Autodesk Inventor part; units mm, degrees
ref_plane "YZ Plane" through (0, 0, 0) normal (1, 0, 0) x (0, 1, 0)
ref_plane "XZ Plane" through (0, 0, 0) normal (0, 1, 0) x (-1, 0, 0)
ref_plane "XY Plane" through (0, 0, 0) normal (0, 0, 1) x (1, 0, 0)
sketch "Sketch1" plane through (0, 0, 0) normal (0, 0, 1) x (1, 0, 0)
  line L0 (-9, -10) -> (9, -10)
  line L1 (9, -10) -> (9, 10)
  line L2 (9, 10) -> (-9, 10)
  line L3 (-9, 10) -> (-9, -10)
  line L4 (-9, -10) -> (9, 10) construction
  line L5 (9, -10) -> (-9, 10) construction
  point P0 (0, 0)
  dimension "d0" = 18
  dimension "d1" = 20
extrude "Plate1" add sketch "Sketch1" along normal blind 2
sketch "Sketch2" plane through (9, -8.1451, -0.7479) normal (0, -0.9274452, 0.3739592) x (1, 0, 0)
  line L0 (-18, 0) -> (0, 0)
  line L1 (0, 0) -> (0, 12)
  line L2 (0, 12) -> (-18, 12)
  line L3 (-18, 12) -> (-18, 0)
edge flange "Flange1" height 12 angle 111.96 thickness 2 bend radius 2 thickness toward (0, -0.9274452, 0.3739592) relief tear relief width 2 relief depth 1 edges at (0, -10, 2) wall of the first edge with corners at (-9, -8.1451, -0.7479) (9, -8.1451, -0.7479) (9, -3.6576, 10.3814) (-9, -3.6576, 10.3814)
bend "Bend1"
corner "Corner1"
chamfer "Corner Chamfer1" distance 2 angle 45 4 edges at (-9, 10, 1) (9, 10, 1) (-9, -4.585, 10.7554) (9, -4.585, 10.7554)
equation "\"d3\" = BendReliefWidth"
equation "\"d4\" = BendReliefDepth"
equation "\"d5\" = MinimumRemnant"
equation "\"d6\" = BendRadius"
equation "\"d9\" = BendRadius"
equation "\"d10\" = CornerReliefSize"
equation "\"d11\" = GapSize"
equation "\"d12\" = JacobiRadiusSize"
equation "\"BendRadius\" = Thickness"
equation "\"BendReliefWidth\" = Thickness"
equation "\"BendReliefDepth\" = 0.5 * Thickness"
equation "\"CornerReliefSize\" = 4 * Thickness"
equation "\"MinimumRemnant\" = 2 * Thickness"
equation "\"TransitionRadius\" = BendRadius"
equation "\"JacobiRadiusSize\" = BendRadius"
equation "\"GapSize\" = Thickness"
equation "\"d2\" = BendRadius"
Here's how the part is built. I have some questions about the finished solid (model axes, mm). A direction names the side the tool comes from. Round coordinates to 2 decimals unless told otherwise and drop trailing zeros. Order: outer loops, then holes, each group sorted by start corner. A loop starts at its lowest first (then second) coordinate and runs counter-clockwise, first axis right, second up. Notation, with made-up numbers: M 81,77.25 L 137,77.25 A20 cw 137,83.25 Z; hole C -25.75,78.25 d5. An arc over 180 degrees is marked long. Answer in a Markdown table with one row per item.
Item 1: I'm going to push a flat-ended pin straight in: pin 1 (2 mm diameter, centred on x = -4.5, y = -0.5, fed in from +Z). Where does the tip first touch, or does it pass through?
A:
| item | result |
|---|---|
| pin 1 | stops at z = 2 |
Item 2: Thinking about a two-plate mould opening in Z: for faces 3 (the face through (0, 3, 0)), 4 (the face through (0.1, -4.57, 10.75)), 5 (the face through (0.126, -5.747, 2.904)), which applies, +Z half, -Z half, draft (parallel to the pull), parting line (faces both ways), or undercut?
A:
| item | result |
|---|---|
| face 3 | -Z half |
| face 4 | +Z half |
| face 5 | undercut |
Item 3: Imagine slicing it at A-A, the plane x = -1.25. Write out the boundary of the cut face in (y, z), and give its area (3 significant figures).
A:
| item | result |
|---|---|
| outline | M -7.78,5.5 A4 ccw -4.07,0 L 10,0 L 10,2 L -4.07,2 A2 cw -5.93,4.75 L -3.66,10.38 L -5.51,11.13 Z |
| area | 52.0 mm2 |
Item 4: Imagine slicing it at D-D, the plane y = 8.25. Write out the boundary of the cut face in (x, z), and give its area (3 significant figures).
A:
| item | result |
|---|---|
| outline | M -8.75,0 L 8.75,0 L 8.75,2 L -8.75,2 Z |
| area | 35.0 mm2 |
Item 5: Imagine slicing it at C-C, the plane z = 8.75. Write out the boundary of the cut face in (x, y), and give its area (3 significant figures).
A:
| item | result |
|---|---|
| outline | M -9,-6.47 L 9,-6.47 L 9,-4.96 L 8.76,-4.32 L -8.76,-4.32 L -9,-4.96 Z |
| area | 38.7 mm2 |
Item 6: Imagine slicing it at B-B, the plane y = -4.75. Write out the boundary of the cut face in (x, z).
A:
| item | result |
|---|---|
| outline | M -9,0.06 L 9,0.06 L 9,2.12 L -9,2.12 Z; M -9,7.67 L 9,7.67 L 9,8.67 L 7,10.82 L -7,10.82 L -9,8.67 Z |
Item 7: For faces 1 (the face through (0.126, -4.809, 7.525)), 2 (the face through (-9, -1.3, 1.6)), which set-ups out of +Z, -Z, +X, -X, +Y, -Y let a thin tool reach every point of the face, with its end or its side?
A:
| item | result |
|---|---|
| face 1 | +X, -X, +Y |
| face 2 | +Z, -Z, -X, +Y, -Y |
Item 8: If I drill on L1, parallel to Z at x = -5.25, y = -4.5; L2, parallel to Z at x = 4, y = 5; L3, parallel to Y at x = -5.25, z = 4, over which ranges is the centre line in solid material (lowest first)? Write a range as from..to.
A:
| item | result |
|---|---|
| L1 | z = 0.02..2.05, 8.29..10.72 |
| L2 | z = 0..2 |
| L3 | y = -8.07..-6.07 |
